```python
from build123d import *

# Parameters (mm, degrees)
SKETCH2_W           = 112
SKETCH2_H           = 80
SKETCH2_W_2         = 20
SKETCH2_H_2         = 3
SKETCH2_W_3         = 3
SKETCH2_H_3         = 15
BOSS_EXTRUDE1_DEPTH = 3


with BuildPart() as part:
    # Sketch2 → Boss-Extrude1 (new body)
    with BuildSketch(Plane.XY):
        Rectangle(SKETCH2_W, SKETCH2_H)
        with Locations((-35, -41.5)):
            Rectangle(SKETCH2_W_2, SKETCH2_H_2)
        with Locations((0, -41.5)):
            Rectangle(SKETCH2_W_2, SKETCH2_H_2)
        with Locations((35, -41.5)):
            Rectangle(SKETCH2_W_2, SKETCH2_H_2)
        with Locations((57.5, -30)):
            Rectangle(SKETCH2_W_3, SKETCH2_H_3)
        with Locations((-57.5, -30)):
            Rectangle(SKETCH2_W_3, SKETCH2_H_3)
        with Locations((-57.5, 0)):
            Rectangle(SKETCH2_W_3, SKETCH2_H_3)
        with Locations((57.5, 0)):
            Rectangle(SKETCH2_W_3, SKETCH2_H_3)
        with Locations((-57.5, 30)):
            Rectangle(SKETCH2_W_3, SKETCH2_H_3)
        with Locations((57.5, 30)):
            Rectangle(SKETCH2_W_3, SKETCH2_H_3)
    extrude(amount=BOSS_EXTRUDE1_DEPTH)


solid = part.part
```
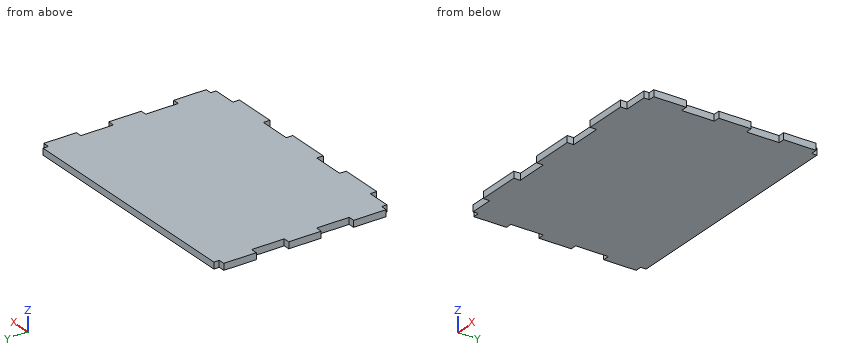
CAD build for the part. Positions are in the model's coordinates, mm. Coordinates: 2 decimals unless noted, no trailing zeros. Write each loop counter-clockwise with the first axis right and the second up, starting at its lowest first coordinate (ties: lowest second). Pieces come first, ordered by that corner, then holes. Notation, with made-up numbers: (24, -4) -> (60, -4) arc R15 cw to (60, 1) -> close; hole circle Ø5 at (41.5, 33.5). An arc over 180 degrees is marked (long way). Use CSV: the item, a comma, the result in double quotes. Start each with the question number.
Item 1: Band-saw the part on A-A, the plane x = 15. Write the cut outline in (y, z).
Item 2: Wall check: probe 1 along Y at (x, z) = (-50, 0.65); probe 2 along X at (y, z) = (-21, 2.5). Give the ranges that are in metal, low to high.
Item 3: Drop flat-ended pins along their axis: P1, Ø1.5, axis at y = -12.5, z = 1, coming from the -X side; P2, Ø0.8, axis at y = 38.5, z = 2, coming from the +X side; P3, Ø0.9, axis at y = -41, z = 1, coming from the +X side. Give the stop position or say it passes through.
Item 4: Band-saw the part on B-B, the plane y = 21. Write the cut outline in (x, z), plus the area to 3 significant figures.
Response values:
1,outline,"(-40, 0) -> (40, 0) -> (40, 3) -> (-40, 3) -> close"
2,probe 1,"y = -40 to 40"
2,probe 2,"x = -56 to 56"
3,P1,"stops at x = -56"
3,P2,"stops at x = 56"
3,P3,"stops at x = 45"
4,outline,"(-56, 0) -> (56, 0) -> (56, 3) -> (-56, 3) -> close"
4,area,"336 mm2"
